For this review, take the finished solid that the model builds, in its own axes (mm). A direction names the side the tool comes from. Coordinates: 2 decimals unless noted, no trailing zeros. Order: outer loops, then holes, each group sorted by start corner. A loop starts at its lowest first (then second) coordinate and runs counter-clockwise, first axis right, second up. Notation, with made-up numbers: (36, -30.75) - (88, -30.75) arc R30 cw to (88, -3.75) - close; hole circle Ø1 at (66.5, 9). An arc over 180 degrees is marked (long way). One line per item, written item: value. Start each with the question number.
(1) To check wall thickness, follow line 1 along Z through (x, y) = (-60, 17.5); line 2 along X through (y, z) = (10.75, -12.5); line 3 along Z through (x, y) = (44.5, 11.5). State the ranges of each line that lie inside material, in increasing order.
(2) Consider section A-A on x = -114. Write out the cut boundary in (y, z).
(3) Consider section B-B on z = 50.5. Write out the cut boundary in (x, y), then the cut area to 4 significant figures.
(4) For faces 4 (the cylindrical face through (152.986, 10.126, -74.297)), 5 (the flat face through (-56, 17, 2)), 6 (the conical face through (-3.01, 24.16, -35.39)), 7 (the cylindrical face through (-155.78, 22.03, 77.16)), 8 (the conical face through (-155.195, 24.84, 76.555)), list the 3-axis set-ups (+Z, -Z, +X, -X, +Y, -Y) from which the entire face can be reached by the end or side of a thin tool; tool diameter is ignored.
(5) Consider section C-C on y = 5. Count the separate pieces of the cut face and the enclosed holes in it, then the cut area to 3 significant figures.
(6) Mouldability with a two-part tool opening along Z and no side actions: class faces 1 (the conical face through (64.45, 19.54, -0.2)), 2 (the conical face through (152.398, 0.16, 73.696)), 3 (the conical face through (-152.398, 0.16, -73.696)) as released by +Z, released by -Z, zero draft, split by the parting line, or undercut.
(7) Clearance check with flat-ended pins moving along their axes: pin 1 (4.5 mm diameter, centred on x = -89.235, z = 24.765, fed in from -Y); pin 2 (5 mm diameter, centred on y = 10.5, z = -3, fed in from +X); pin 3 (3 mm diameter, centred on x = 45, z = 70, fed in from -Y); pin 4 (3 mm diameter, centred on y = 9.5, z = -30, fed in from -X). State where each tip first meets the part, or that it passes through.
```python
from build123d import *

# Parameters (mm, degrees)
SKETCH1_W                                            = 318
SKETCH1_H                                            = 160
BOSS_EXTRUDE1_DEPTH                                  = 25
SKETCH2_R                                            = 28.5
CUT_EXTRUDE1_DEPTH                                   = 180.738699228
CUT_EXTRUDE2_DEPTH                                   = 180.738699228
CUT_EXTRUDE2_DEPTH_BACK                              = 180.738699228
SKETCH4_R                                            = 9.55
CHAMFER1_SIZE                                        = 0.5
FILLET1_R                                            = 20
M8_CLEARANCE_HOLE1_D                                 = 9
M6X1_0_TAPPED_HOLE1_D                                = 5
SKETCH13_R                                           = 13.411040831
SKETCH13_R_2                                         = 14.724493856
BOSS_EXTRUDE3_DEPTH                                  = 8
CSK_FOR_5_16_FLAT_HEAD_SOCKET_CAP_SCREW1_D           = 8.4328
CSK_FOR_5_16_FLAT_HEAD_SOCKET_CAP_SCREW1_CSINK_D     = 18.4009792
CSK_FOR_5_16_FLAT_HEAD_SOCKET_CAP_SCREW1_CSINK_ANGLE = 82
BOSS_EXTRUDE4_DEPTH                                  = 6
CUT_EXTRUDE3_DEPTH                                   = 186.067555233
CHAMFER4_SIZE                                        = 1
M6X1_0_TAPPED_HOLE2_D                                = 5
M6X1_0_TAPPED_HOLE2_DEPTH                            = 15
M6X1_0_TAPPED_HOLE2_TIP                              = 1.502151548


with BuildPart() as part:
    # Sketch1 → Boss-Extrude1 (new body)
    with BuildSketch(Plane(origin=(0, 0, 0), x_dir=(1, 0, 0), z_dir=(0, 1, 0))):
        Rectangle(SKETCH1_W, SKETCH1_H)
    extrude(amount=BOSS_EXTRUDE1_DEPTH)

    # Sketch2 → Cut-Extrude1 (cut, through all)
    with BuildSketch(Plane(origin=(0, 25, 0), x_dir=(1, 0, 0), z_dir=(0, 1, 0))):
        with Locations(Location((-114, 0, 0), (0, 0, 270))):
            Circle(SKETCH2_R)
        with Locations(Location((114, 0, 0), (0, 0, 270))):
            Circle(SKETCH2_R)
    extrude(amount=-CUT_EXTRUDE1_DEPTH, mode=Mode.SUBTRACT)

    # Sketch4 → Cut-Extrude2 (cut, two sides: drawn at the far end of the back side and taken through both)
    with BuildSketch(Plane(origin=(0, 25, 0), x_dir=(1, 0, 0), z_dir=(0, 1, 0)).offset(-CUT_EXTRUDE2_DEPTH_BACK)):
        with Locations(Location((-60, 0, 0), (0, 0, 270))):
            Circle(SKETCH4_R)
        with Locations(Location((60, 0, 0), (0, 0, 270))):
            Circle(SKETCH4_R)
    extrude(amount=CUT_EXTRUDE2_DEPTH + CUT_EXTRUDE2_DEPTH_BACK, mode=Mode.SUBTRACT)

    # Chamfer1
    chamfer1_edges = [part.edges().sort_by_distance(p)[0] for p in [
        (-114, 0, -28.5),
        (-114, 25, -28.5),
        (114, 0, -28.5),
        (114, 25, -28.5),
        (-60, 0, -9.55),
        (-60, 25, -9.55),
        (60, 0, -9.55),
        (60, 25, -9.55),
    ]]
    chamfer(chamfer1_edges, length=CHAMFER1_SIZE)

    # Fillet1
    fillet1_edges = [part.edges().sort_by_distance(p)[0] for p in [
        (159, 12.5, 80),
        (-159, 12.5, 80),
        (-159, 12.5, -80),
        (159, 12.5, -80),
    ]]
    fillet(fillet1_edges, radius=FILLET1_R)

    # M8 Clearance Hole1 (through all)
    with Locations(Plane.XZ):
        with Locations((-139, -60), (-139, 60), (139, -60), (139, 60)):
            Hole(M8_CLEARANCE_HOLE1_D / 2)

    # M6x1.0 Tapped Hole1 (through all)
    with Locations(Plane(origin=(0, 0, 0), x_dir=(-1, 0, 0), z_dir=(0, -1, 0))):
        with Locations((138.765, -24.765), (89.235, -24.765), (89.235, 24.765), (138.765, 24.765), (-89.235, -24.765), (-138.765, -24.765), (-89.235, 24.765), (-138.765, 24.765)):
            Hole(M6X1_0_TAPPED_HOLE1_D / 2)

    # Sketch13 → Boss-Extrude3 (add)
    with BuildSketch(Plane(origin=(0, 25, 0), x_dir=(1, 0, 0), z_dir=(0, 1, 0))):
        with Locations((60, 0)):
            Circle(SKETCH13_R)
        with Locations((-60, 0)):
            Circle(SKETCH13_R_2)
    extrude(amount=-BOSS_EXTRUDE3_DEPTH)

    # CSK for 5/16 Flat Head Socket Cap Screw1 (through all)
    with Locations(Plane(origin=(0, 25, 0), x_dir=(1, 0, 0), z_dir=(0, 1, 0))):
        with Locations((60, 0), (-60, 0)):
            CounterSinkHole(CSK_FOR_5_16_FLAT_HEAD_SOCKET_CAP_SCREW1_D / 2, CSK_FOR_5_16_FLAT_HEAD_SOCKET_CAP_SCREW1_CSINK_D / 2, counter_sink_angle=CSK_FOR_5_16_FLAT_HEAD_SOCKET_CAP_SCREW1_CSINK_ANGLE)

    # Sketch16 → Boss-Extrude4 (add)
    with BuildSketch(Plane.XZ.offset(-25)):
        with BuildLine():
            Line((163, -60), (163, 60))
            ThreePointArc((163, 60), (155.970562748, 76.970562748), (139, 84))
            Line((139, 84), (-139, 84))
            ThreePointArc((-139, 84), (-155.970562748, 76.970562748), (-163, 60))
            Line((-163, 60), (-163, -60))
            ThreePointArc((-163, -60), (-155.970562748, -76.970562748), (-139, -84))
            Line((-139, -84), (139, -84))
            ThreePointArc((139, -84), (155.970562748, -76.970562748), (163, -60))
        make_face()
        with BuildLine():
            Line((159, 60), (159, -60))
            ThreePointArc((159, -60), (153.142135624, -74.142135624), (139, -80))
            Line((139, -80), (-139, -80))
            ThreePointArc((-139, -80), (-153.142135624, -74.142135624), (-159, -60))
            Line((-159, -60), (-159, 60))
            ThreePointArc((-159, 60), (-153.142135624, 74.142135624), (-139, 80))
            Line((-139, 80), (139, 80))
            ThreePointArc((139, 80), (153.142135624, 74.142135624), (159, 60))
        make_face(mode=Mode.SUBTRACT)
    extrude(amount=BOSS_EXTRUDE4_DEPTH)

    # Sketch17 → Cut-Extrude3 (cut, through all)
    with BuildSketch(Plane.XZ):
        with BuildLine():
            Line((-60, -18.184097247), (-20, -18.184097247))
            ThreePointArc((-20, -18.184097247), (-3.164859361, -35.019237886), (-20, -51.854378525))
            Line((-20, -51.854378525), (-60, -51.854378525))
            ThreePointArc((-60, -51.854378525), (-76.835140639, -35.019237886), (-60, -18.184097247))
        make_face()
    extrude(amount=-CUT_EXTRUDE3_DEPTH, mode=Mode.SUBTRACT)

    # Chamfer4
    chamfer4_edges = [part.edges().sort_by_distance(p)[0] for p in [
        (-134.5, 0, 60),
        (-134.5, 25, 60),
        (-134.5, 0, -60),
        (-134.5, 25, -60),
        (155.970562748, 19, -76.970562748),
        (163, 19, 0),
        (155.970562748, 19, 76.970562748),
        (0, 19, 84),
        (-155.970562748, 19, 76.970562748),
        (-163, 19, 0),
        (-155.970562748, 19, -76.970562748),
        (0, 19, -84),
        (155.970562748, 25, -76.970562748),
        (163, 25, 0),
        (155.970562748, 25, 76.970562748),
        (0, 25, 84),
        (-155.970562748, 25, 76.970562748),
        (-163, 25, 0),
        (-155.970562748, 25, -76.970562748),
        (0, 25, -84),
        (-76.835140639, 25, -35.019237886),
        (-40, 25, -18.184097247),
        (-3.164859361, 25, -35.019237886),
        (-40, 25, -51.854378525),
        (-76.835140639, 0, -35.019237886),
        (-40, 0, -51.854378525),
        (-3.164859361, 0, -35.019237886),
        (-40, 0, -18.184097247),
        (159, 0, 0),
        (0, 0, 80),
        (-159, 0, 0),
        (0, 0, -80),
        (-153.142135624, 0, 74.142135624),
        (-153.142135624, 0, -74.142135624),
        (153.142135624, 0, -74.142135624),
        (153.142135624, 0, 74.142135624),
        (143.5, 0, 60),
        (143.5, 25, 60),
        (143.5, 0, -60),
        (143.5, 25, -60),
    ]]
    chamfer(chamfer4_edges, length=CHAMFER4_SIZE)

    # M6x1.0 Tapped Hole2
    with Locations(Plane(origin=(0, 0, 0), x_dir=(-1, 0, 0), z_dir=(0, -1, 0))):
        with Locations((-75, 70), (-45, 70), (-105, 70), (-15, 70), (15, 70), (45, 70), (75, 70), (105, 70), (-105, -70), (-75, -70), (-45, -70), (-15, -70), (15, -70), (45, -70), (75, -70), (105, -70)):
            Hole(M6X1_0_TAPPED_HOLE2_D / 2, depth=M6X1_0_TAPPED_HOLE2_DEPTH)
            with Locations((0, 0, -(M6X1_0_TAPPED_HOLE2_DEPTH + M6X1_0_TAPPED_HOLE2_TIP / 2))):  # 118° drill point
                Cone(0, M6X1_0_TAPPED_HOLE2_D / 2, M6X1_0_TAPPED_HOLE2_TIP, mode=Mode.SUBTRACT)


solid = part.part
```
Geometry check:
1. line 1: z = -80 to -51.85, -18.18 to -4.22, 4.22 to 80
1. line 2: x = -159 to -139.61, -88.39 to 88.39, 139.61 to 159
1. line 3: z = -80 to -72.45, -67.55 to 67.55, 72.45 to 80
2. outline: (0, -79) - (1, -80) - (19, -80) - (19, -83) - (20, -84) - (24, -84) - (25, -83) - (25, -29) - (24.5, -28.5) - (0.5, -28.5) - (0, -29) - close; (0, 29) - (0.5, 28.5) - (24.5, 28.5) - (25, 29) - (25, 83) - (24, 84) - (20, 84) - (19, 83) - (19, 80) - (1, 80) - (0, 79) - close
3. outline: (-163, 20) - (-162, 19) - (-159, 19) - (-159, 1) - (-158, 0) - (158, 0) - (159, 1) - (159, 19) - (162, 19) - (163, 20) - (163, 24) - (162, 25) - (-162, 25) - (-163, 24) - close
3. area: 7,995 mm^2
4. face 4: -Z, +X, -Y
4. face 5: -Y
4. face 6: +Y
4. face 7: +Z, -X, +Y, -Y
4. face 8: +Z, -X, +Y
5. separate pieces: 1
5. enclosed holes: 33
5. area: 41,900 mm^2
6. face 1: undercut
6. face 2: released by +Z
6. face 3: released by -Z
7. pin 1: passes through
7. pin 2: stops at x = 159
7. pin 3: stops at y = 15.6
7. pin 4: stops at x = -159
